CAD build for the part. Positions are in the model's coordinates, mm. A direction names the side the tool comes from. Give positions to 0.01 mm unless a question says otherwise; leave off trailing zeros. Write each loop counter-clockwise with the first axis right and the second up, starting at its lowest first coordinate (ties: lowest second). Pieces come first, ordered by that corner, then holes. Notation, with made-up numbers: (15.25, 7) -> (52.25, 7) arc R18 ccw to (52.25, 29) -> close; hole circle Ø4 at (-21.75, 26.25). An arc over 180 degrees is marked (long way). Answer as a JSON object with one key per item and string values.
Autodesk Inventor part; units mm, degrees
ref_plane "YZ Plane" through (0, 0, 0) normal (1, 0, 0) x (0, 1, 0)
ref_plane "XZ Plane" through (0, 0, 0) normal (0, 1, 0) x (-1, 0, 0)
ref_plane "XY Plane" through (0, 0, 0) normal (0, 0, 1) x (1, 0, 0)
sketch "Sketch1" plane through (0, 0, 0) normal (0, 1, 0) x (-1, 0, 0)
  line L0 (-22.5, 20) -> (22.5, 20)
  line L1 (22.5, 20) -> (22.5, -20)
  line L2 (22.5, -20) -> (-22.5, -20)
  line L3 (-22.5, -20) -> (-22.5, 20)
  line L4 (-22.5, 20) -> (22.5, -20) construction
  line L5 (22.5, 20) -> (-22.5, -20) construction
  arc A0 (22.5, -20) -> (22.5, 20) centre (22.5, 0) ccw
  point P0 (0, 0)
  dimension "d0" = 45
  dimension "d1" = 40
  dimension "d2" = 20
extrude "Extrusion1" add sketch "Sketch1" along normal blind 3
sketch "Sketch2" plane through (0, 3, 0) normal (0, 1, 0) x (1, 0, 0)
  arc A0 (-22.5, 20) -> (-22.5, -20) centre (-22.5, 0) ccw construction
  line L0 (-42.5, 0) -> (-27.5, 0) construction
  point P0 (0, 0)
  dimension "d5" = 15
hole "Hole1" at (-27.5, 3, 0) direction (0, -1, 0) diameter 13 end through all
sketch "Sketch4" plane through (0, 0, 0) normal (0, -1, 0) x (1, 0, 0)
  line L0 (22.5, 20) -> (22.5, -20) construction
  line L1 (22.5, 0) -> (12.5, 0) construction
  line L2 (11, -7.5) -> (14, -7.5)
  line L3 (14, -7.5) -> (14, 7.5)
  line L4 (14, 7.5) -> (11, 7.5)
  line L5 (11, 7.5) -> (11, -7.5)
  line L6 (11, -7.5) -> (14, 7.5) construction
  line L7 (14, -7.5) -> (11, 7.5) construction
  point P0 (0, 0)
  dimension "d17" = 10
  dimension "d18" = 3
  dimension "d19" = 15
extrude "Extrusion3" cut sketch "Sketch4" against normal blind 10
fillet "Fillet1" radius 3 2 edges at (22.5, 1.5, -20) (22.5, 1.5, 20)
properties part number "sample_mount"
1) Slice it at D-D (z = 16). List the corners of the cut face in (x, y), then the cut area to 3 significant figures.
Model answer:
{"outline": "(-34.5, 0) -> (22.5, 0) -> (22.5, 3) -> (-34.5, 3) -> close", "area": "171 mm2"}
2) Slice it at A-A (y = 2.3). List the corners of the cut face in (x, z).
Model answer:
{"outline": "(-22.5, -20) -> (19.5, -20) arc R3 ccw to (22.5, -17) -> (22.5, 17) arc R3 ccw to (19.5, 20) -> (-22.5, 20) arc R20 ccw to start; hole circle Ø13 at (-27.5, 0); hole (11, -7.5) -> (14, -7.5) -> (14, 7.5) -> (11, 7.5) -> close"}
3) Mould opens along Z. For faces 1 (the flat face through (-2, 1, -20)), 2 (the cylindrical face through (-33.945, 1.479, -0.846)), 3 (the flat face through (-10, 0, 0)), 4 (the flat face through (11, 1, 0)) say: released by +Z, released by -Z, zero draft, split by the parting line, or undercut.
Model answer:
{"face 1": "released by -Z", "face 2": "undercut", "face 3": "zero draft", "face 4": "undercut"}
4) 3-axis set-ups, long thin cutter, end or side, ignore diameter. For faces 5 (the flat face through (-1, 1, 20)), 6 (the flat face through (12, 1, -7.5)): which of +Z, -Z, +X, -X, +Y, -Y reach the whole face in a straight line?
Model answer:
{"face 5": "+Z, +X, -X, +Y, -Y", "face 6": "+Y, -Y"}
5) Wall check: probe 1 along X at (y, z) = (1.25, 0); probe 2 along X at (y, z) = (0.4, -5.5); probe 3 along Z at (x, y) = (12, 1.4). Give the ranges that are in metal, low to high.
Model answer:
{"probe 1": "x = -42.5 to -34, -21 to 11, 14 to 22.5", "probe 2": "x = -41.73 to -30.96, -24.04 to 11, 14 to 22.5", "probe 3": "z = -20 to -7.5, 7.5 to 20"}
6) Pin check, flat tips, straight feed: pin 1 (0.9 mm diameter, centred on y = 2, z = 3, fed in from -X); pin 2 (1.5 mm diameter, centred on y = 0.5, z = 9, fed in from -X). Stop position of each tip, or through.
Model answer:
{"pin 1": "stops at x = -42.34", "pin 2": "stops at x = -40.72"}
7) Slice it at B-B (x = -27.5). List the corners of the cut face in (y, z), then the cut area to 3 significant figures.
Model answer:
{"outline": "(0, -19.36) -> (3, -19.36) -> (3, -6.5) -> (0, -6.5) -> close; (0, 6.5) -> (3, 6.5) -> (3, 19.36) -> (0, 19.36) -> close", "area": "77.2 mm2"}
8) Slice it at C-C (z = 2.5). List the corners of the cut face in (x, y), then the cut area to 3 significant figures.
Model answer:
{"outline": "(-42.34, 0) -> (-33.5, 0) -> (-33.5, 3) -> (-42.34, 3) -> close; (-21.5, 0) -> (11, 0) -> (11, 3) -> (-21.5, 3) -> close; (14, 0) -> (22.5, 0) -> (22.5, 3) -> (14, 3) -> close", "area": "150 mm2"}
